from build123d import *

# Parameters (mm, degrees)
CROQUIS1_W               = 90
CROQUIS1_H               = 76.2
CROQUIS1_R               = 4
SALIENTE_EXTRUIR1_DEPTH  = 0.47625
CROQUIS1_2_W             = 90
CROQUIS1_2_H             = 76.2
CROQUIS1_2_R             = 4
SALIENTE_EXTRUIR2_DEPTH  = 4.7625
CROQUIS3_W               = 90
CROQUIS3_H               = 4.7625
SALIENTE_EXTRUIR3_DEPTH  = 4.445
CROQUIS5_W               = 90
CROQUIS5_H               = 4.7625
SALIENTE_EXTRUIR4_DEPTH  = 4.445
CROQUIS6_W               = 4.7625
CROQUIS6_H               = 85.09
SALIENTE_EXTRUIR5_DEPTH  = 5
CROQUIS7_W               = 4.7625
CROQUIS7_H               = 85.09
SALIENTE_EXTRUIR6_DEPTH  = 5
CROQUIS8_W               = 100
CROQUIS8_H               = 4.7625
SALIENTE_EXTRUIR7_DEPTH  = 4.445
CROQUIS9_W               = 100
CROQUIS9_H               = 4.7625
SALIENTE_EXTRUIR8_DEPTH  = 4.445
CROQUIS10_W              = 4.7625
CROQUIS10_H              = 93.98
SALIENTE_EXTRUIR9_DEPTH  = 5
CROQUIS12_W              = 4.7625
CROQUIS12_H              = 93.98
SALIENTE_EXTRUIR10_DEPTH = 5
SKETCH1_R                = 8.75
CUT_EXTRUDE1_DEPTH       = 10
SKETCH2_R                = 2
CUT_EXTRUDE2_DEPTH       = 10
SKETCH3_R                = 1.5
CUT_EXTRUDE3_DEPTH       = 10
SKETCH4_R                = 2
CUT_EXTRUDE4_DEPTH       = 10


with BuildPart() as part:
    # Croquis1 → Saliente-Extruir1 (new body)
    with BuildSketch(Plane.XY):
        with Locations((45, 38.1)):
            Rectangle(CROQUIS1_W, CROQUIS1_H)
        with Locations((45, 38.1)):
            Circle(CROQUIS1_R, mode=Mode.SUBTRACT)
        with Locations((10, 9.95)):
            Circle(CROQUIS1_R, mode=Mode.SUBTRACT)
        with Locations((10, 66.25)):
            Circle(CROQUIS1_R, mode=Mode.SUBTRACT)
        with Locations((80, 66.25)):
            Circle(CROQUIS1_R, mode=Mode.SUBTRACT)
        with Locations((80, 9.95)):
            Circle(CROQUIS1_R, mode=Mode.SUBTRACT)
        with Locations((45, 66.25)):
            Circle(CROQUIS1_R, mode=Mode.SUBTRACT)
        with Locations((10, 38.1)):
            Circle(CROQUIS1_R, mode=Mode.SUBTRACT)
        with Locations((80, 38.1)):
            Circle(CROQUIS1_R, mode=Mode.SUBTRACT)
        with Locations((45, 9.95)):
            Circle(CROQUIS1_R, mode=Mode.SUBTRACT)
    extrude(amount=SALIENTE_EXTRUIR1_DEPTH)

    # Croquis1<2> → Saliente-Extruir2 (add)
    with BuildSketch(Plane.XY):
        with Locations((45, 38.1)):
            Rectangle(CROQUIS1_2_W, CROQUIS1_2_H)
        with Locations((45, 38.1)):
            Circle(CROQUIS1_2_R, mode=Mode.SUBTRACT)
        with Locations((10, 9.95)):
            Circle(CROQUIS1_2_R, mode=Mode.SUBTRACT)
        with Locations((10, 66.25)):
            Circle(CROQUIS1_2_R, mode=Mode.SUBTRACT)
        with Locations((80, 66.25)):
            Circle(CROQUIS1_2_R, mode=Mode.SUBTRACT)
        with Locations((80, 9.95)):
            Circle(CROQUIS1_2_R, mode=Mode.SUBTRACT)
        with Locations((45, 66.25)):
            Circle(CROQUIS1_2_R, mode=Mode.SUBTRACT)
        with Locations((10, 38.1)):
            Circle(CROQUIS1_2_R, mode=Mode.SUBTRACT)
        with Locations((80, 38.1)):
            Circle(CROQUIS1_2_R, mode=Mode.SUBTRACT)
        with Locations((45, 9.95)):
            Circle(CROQUIS1_2_R, mode=Mode.SUBTRACT)
    extrude(amount=SALIENTE_EXTRUIR2_DEPTH)

    # Croquis3 → Saliente-Extruir3 (add)
    with BuildSketch(Plane.XZ):
        with Locations((45, 2.38125)):
            Rectangle(CROQUIS3_W, CROQUIS3_H)
    extrude(amount=SALIENTE_EXTRUIR3_DEPTH)

    # Croquis5 → Saliente-Extruir4 (add)
    with BuildSketch(Plane(origin=(0, 76.2, 0), x_dir=(1, 0, 0), z_dir=(0, 1, 0))):
        with Locations((45, -2.38125)):
            Rectangle(CROQUIS5_W, CROQUIS5_H)
    extrude(amount=SALIENTE_EXTRUIR4_DEPTH)

    # Croquis6 → Saliente-Extruir5 (add)
    with BuildSketch(Plane.ZY):
        with Locations((2.38125, 38.1)):
            Rectangle(CROQUIS6_W, CROQUIS6_H)
    extrude(amount=SALIENTE_EXTRUIR5_DEPTH)

    # Croquis7 → Saliente-Extruir6 (add)
    with BuildSketch(Plane(origin=(90, 0, 0), x_dir=(0, 0, -1), z_dir=(1, 0, 0))):
        with Locations((-2.38125, 38.1)):
            Rectangle(CROQUIS7_W, CROQUIS7_H)
    extrude(amount=SALIENTE_EXTRUIR6_DEPTH)

    # Croquis8 → Saliente-Extruir7 (add)
    with BuildSketch(Plane.XZ.offset(4.445)):
        with Locations((45, 2.38125)):
            Rectangle(CROQUIS8_W, CROQUIS8_H)
    extrude(amount=SALIENTE_EXTRUIR7_DEPTH)

    # Croquis9 → Saliente-Extruir8 (add)
    with BuildSketch(Plane(origin=(0, 80.645, 0), x_dir=(1, 0, 0), z_dir=(0, 1, 0))):
        with Locations((45, -2.38125)):
            Rectangle(CROQUIS9_W, CROQUIS9_H)
    extrude(amount=SALIENTE_EXTRUIR8_DEPTH)

    # Croquis10 → Saliente-Extruir9 (add)
    with BuildSketch(Plane(origin=(95, 0, 0), x_dir=(0, 0, -1), z_dir=(1, 0, 0))):
        with Locations((-2.38125, 38.1)):
            Rectangle(CROQUIS10_W, CROQUIS10_H)
    extrude(amount=SALIENTE_EXTRUIR9_DEPTH)

    # Croquis12 → Saliente-Extruir10 (add)
    with BuildSketch(Plane.ZY.offset(5)):
        with Locations((2.38125, 38.1)):
            Rectangle(CROQUIS12_W, CROQUIS12_H)
    extrude(amount=SALIENTE_EXTRUIR10_DEPTH)

    # Sketch1 → Cut-Extrude1 (cut)
    with BuildSketch(Plane(origin=(0, 0, 0), x_dir=(-1, 0, 0), z_dir=(0, 0, -1))):
        with Locations((-80, 9.95)):
            Circle(SKETCH1_R)
        with Locations((-10, 9.95)):
            Circle(SKETCH1_R)
    extrude(amount=-CUT_EXTRUDE1_DEPTH, mode=Mode.SUBTRACT)

    # Sketch2 → Cut-Extrude2 (cut)
    with BuildSketch(Plane(origin=(0, 0, 0), x_dir=(-1, 0, 0), z_dir=(0, 0, -1))):
        with Locations((-95, 75.09)):
            Circle(SKETCH2_R)
    extrude(amount=-CUT_EXTRUDE2_DEPTH, mode=Mode.SUBTRACT)

    # Sketch3 → Cut-Extrude3 (cut)
    with BuildSketch(Plane.XY.offset(4.7625)):
        with Locations((96, 9.026516715)):
            Circle(SKETCH3_R)
    extrude(amount=-CUT_EXTRUDE3_DEPTH, mode=Mode.SUBTRACT)

    # Sketch4 → Cut-Extrude4 (cut)
    with BuildSketch(Plane(origin=(0, 0, 0), x_dir=(-1, 0, 0), z_dir=(0, 0, -1))):
        with Locations((6, 35.220430455)):
            Circle(SKETCH4_R)
        with Locations((-96, 35.220430455)):
            Circle(SKETCH4_R)
    extrude(amount=-CUT_EXTRUDE4_DEPTH, mode=Mode.SUBTRACT)


solid = part.part
Build history of the part. All positions in model axes, mm. Round coordinates to 2 decimals unless told otherwise and drop trailing zeros. Write each loop counter-clockwise with the first axis right and the second up, starting at its lowest first coordinate (ties: lowest second). Pieces come first, ordered by that corner, then holes. Notation, with made-up numbers: (35.25, 60.25) - (77.25, 60.25) arc R16 cw to (77.25, 90.25) - close; hole circle Ø1 at (87, -22). An arc over 180 degrees is marked (long way). Use CSV: the item, a comma, the result in double quotes.
(1) Wall check: line 1 (Y direction, x = 10, z = 2.25); line 2 (Y direction, x = 45, z = 1.5); line 3 (X direction, y = 10, z = 1.4). Give the ranges that are in metal, low to high.
Response:
line 1,"-8.89 to 1.2, 18.7 to 34.1, 42.1 to 62.25, 70.25 to 85.09"
line 2,"-8.89 to 5.95, 13.95 to 34.1, 42.1 to 62.25, 70.25 to 85.09"
line 3,"-10 to 1.25, 18.75 to 41, 49 to 71.25, 88.75 to 94.86, 97.14 to 100"
(2) Band-saw the part on A-A (y = 75.09). Write the cut outline in (x, z).
Response:
outline,"(-10, 0) - (93, 0) - (93, 4.76) - (-10, 4.76) - close; (97, 0) - (100, 0) - (100, 4.76) - (97, 4.76) - close"
(3) Band-saw the part on D-D (x = 45). Write the cut outline in (y, z), plus the area to 3 significant figures.
Response:
outline,"(-8.89, 0) - (5.95, 0) - (5.95, 4.76) - (-8.89, 4.76) - close; (13.95, 0) - (34.1, 0) - (34.1, 4.76) - (13.95, 4.76) - close; (42.1, 0) - (62.25, 0) - (62.25, 4.76) - (42.1, 4.76) - close; (70.25, 0) - (85.09, 0) - (85.09, 4.76) - (70.25, 4.76) - close"
area,"333 mm²"
(4) Band-saw the part on C-C (z = 3.2). Give the number of separate pieces and of enclosed holes in the cut face, plus the area to 3 significant figures.
Response:
separate pieces,"1"
enclosed holes,"13"
area,"9,460 mm²"
(5) Pin check, flat tip, straight feed: P1, Ø5, axis at x = 96, y = 9.03, coming from the -Z side. Stop position of the tip, or through.
Response:
P1,"z = 0"
(6) Band-saw the part on B-B (x = 80). Write the cut outline in (y, z), plus the area to 3 significant figures.
Response:
outline,"(-8.89, 0) - (1.2, 0) - (1.2, 4.76) - (-8.89, 4.76) - close; (18.7, 0) - (34.1, 0) - (34.1, 4.76) - (18.7, 4.76) - close; (42.1, 0) - (62.25, 0) - (62.25, 4.76) - (42.1, 4.76) - close; (70.25, 0) - (85.09, 0) - (85.09, 4.76) - (70.25, 4.76) - close"
area,"288 mm²"
(7) Mould opens along Y. For faces 1 (the cylindrical face through (76, 38, 2)), 2 (the flat face through (46, -8.89, 2)), 3 (the flat face through (100, 39, 2)) say: pulls with the +Y half, pulls with the -Y half, needs draft (parallel to the pull), parting line crosses it, or undercut.
Response:
face 1,"undercut"
face 2,"pulls with the -Y half"
face 3,"needs draft"
